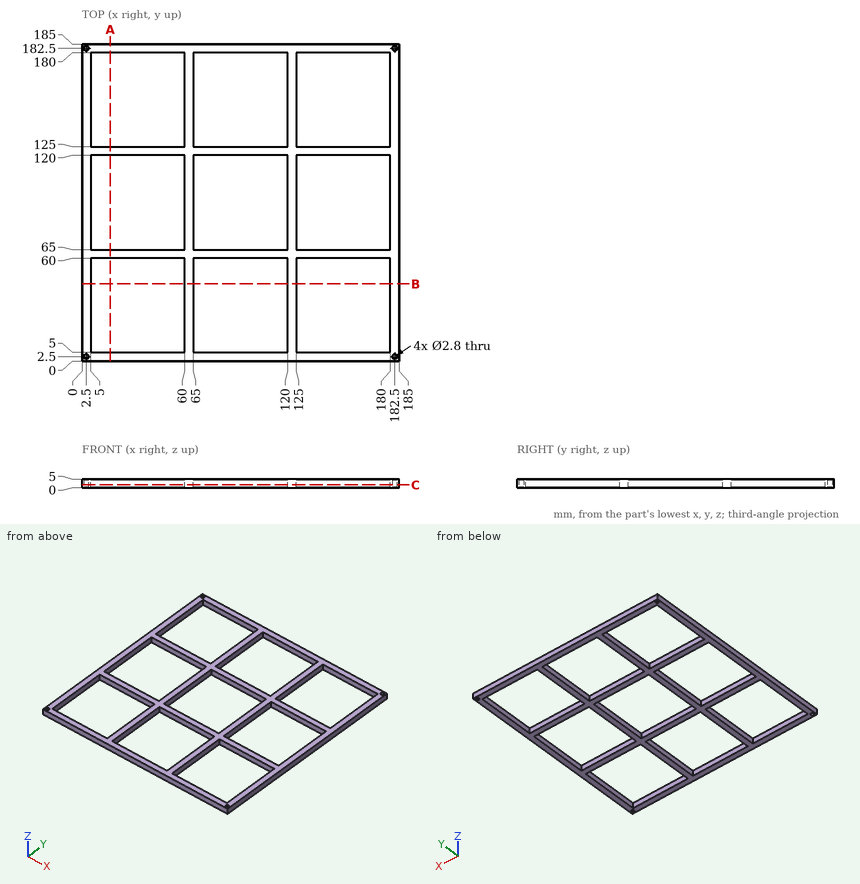
Print and shaded views of the part. All mm, measured from the part's lowest x, y and z. Coordinates: 2 decimals unless noted, no trailing zeros. Order: outer loops, then holes, each group sorted by start corner. A loop starts at its lowest first (then second) coordinate and runs counter-clockwise, first axis right, second up.
(1) Probe L1, parallel to Y at x = 2.5, z = 3.75; L2, parallel to Y at x = 139, z = 1.55. List the from-to ranges inside material, lowest first.
Check sheet entries:
L1: y = 0 to 1.1, 3.9 to 181.1, 183.9 to 185
L2: y = 0 to 5, 60 to 65, 120 to 125, 180 to 185
(2) Slice it at A-A, the plane x = 16.5. Write the cut outline in (y, z).
Check sheet entries:
outline: (0, 0) - (5, 0) - (5, 5) - (0, 5) - close; (60, 0) - (65, 0) - (65, 5) - (60, 5) - close; (120, 0) - (125, 0) - (125, 5) - (120, 5) - close; (180, 0) - (185, 0) - (185, 5) - (180, 5) - close
(3) Pin check, flat tips, straight feed: pin 1 Ø3 at (y, z) = (69.5, 4) entering from -X; pin 2 Ø2.5 at (x, y) = (182.5, 182.5) entering from -Z. Stop position of each tip, or through.
Check sheet entries:
pin 1: stops at x = 0
pin 2: passes through
(4) Slice it at C-C, the plane z = 1.55. State how many separate pieces and enclosed holes the cut face has, and give its area (3 significant figures).
Check sheet entries:
separate pieces: 1
enclosed holes: 13
area: 6,980 mm2
